Can you work these out from the model? Positions are in its coordinate system, mm. Face numbers are marked on the shaded views. A direction names the side the tool comes from. Coordinates: 2 decimals unless noted, no trailing zeros. Order: outer loops, then holes, each group sorted by start corner. A loop starts at its lowest first (then second) coordinate and runs counter-clockwise, first axis right, second up. Notation, with made-up numbers: (-31, 29.5) -> (-17, 29.5) arc R24 ccw to (-17, 47.5) -> close; hole circle Ø4 at (8.25, -23). An arc over 180 degrees is marked (long way). Return JSON: item names as keys, results as strings. Group by question number.
1) For pin 1 (1 mm diameter, centred on x = -7.5, y = -1.5, fed in from +Z); pin 2 (10 mm diameter, centred on x = -8.5, z = 5.5, fed in from -Y); pin 3 (9.5 mm diameter, centred on x = 2, y = 7, fed in from -Z); pin 4 (1 mm diameter, centred on y = 4, z = 8.5, fed in from +X), each with a flat end and sliding along its axis, tell me the tip position at first contact or that it passes through.
2) If I drill on probe 1 along Z at (x, y) = (-5, 11); probe 2 along Y at (x, z) = (0, 17.25); probe 3 along Y at (x, z) = (0, 2) (3 decimals), over which ranges is the centre line in solid material (lowest first)? Write a range as from..to.
3) If we section it at C-C, the plane z = 17.5: Please give me the cut outline in (x, y).
4) Thinking about a two-plate mould opening in X: for the marked faces 1, 2 and 3, which applies, +X half, -X half, draft (parallel to the pull), parting line (faces both ways), or undercut?
5) If we section it at A-A, the plane x = 0: Please give me the cut outline in (y, z) (3 decimals), then the cut area to 3 significant figures.
6) For the marked faces 4 and 5, which set-ups out of +Z, -Z, +X, -X, +Y, -Y let a thin tool reach every point of the face, with its end or its side?
7) If we section it at D-D, the plane y = 10.5: Please give me the cut outline in (x, z).
from build123d import *

# Parameters (mm, degrees)
F0_R     = 12.5
F1_DEPTH = 21.5
F2_R     = 15.85
F2_R_2   = 12.5
F3_DEPTH = 2
F5_D     = 15.75
F5_DEPTH = 23.5
F5_TIP   = 4.7317773748
F6_R     = 10
F7_DEPTH = 17
F8_W     = 1
F8_H     = 1.25


with BuildPart() as f1:
    # F0 (on Top) → F1 (new body)
    with BuildSketch(Plane.XY):
        Circle(F0_R)
    extrude(amount=F1_DEPTH)

    # F2 (on face) → F3 (join)
    with BuildSketch(Plane.XY.offset(21.5)):
        Circle(F2_R)
        Circle(F2_R_2, mode=Mode.SUBTRACT)
        Circle(F2_R_2)
    extrude(amount=F3_DEPTH)

    # F5
    with Locations(Plane.XY.offset(23.5)):
        with Locations((0, 0)):
            Hole(F5_D / 2, depth=F5_DEPTH)
            with Locations((0, 0, -(F5_DEPTH + F5_TIP / 2))):  # 118° drill point
                Cone(0, F5_D / 2, F5_TIP, mode=Mode.SUBTRACT)

    # F6 (on face) → F7 (cut)
    with BuildSketch(Plane.XY.offset(23.5)):
        Circle(F6_R)
    extrude(amount=-F7_DEPTH, mode=Mode.SUBTRACT)

    # F8 (on Front) → F9 (revolve, cut)
    with BuildSketch(Plane.XZ):
        with Locations((-12, 15.375)):
            Rectangle(F8_W, F8_H)
    revolve(axis=Axis((0, 0, 8), (0, 0, 1)), mode=Mode.SUBTRACT)


solid = f1.part
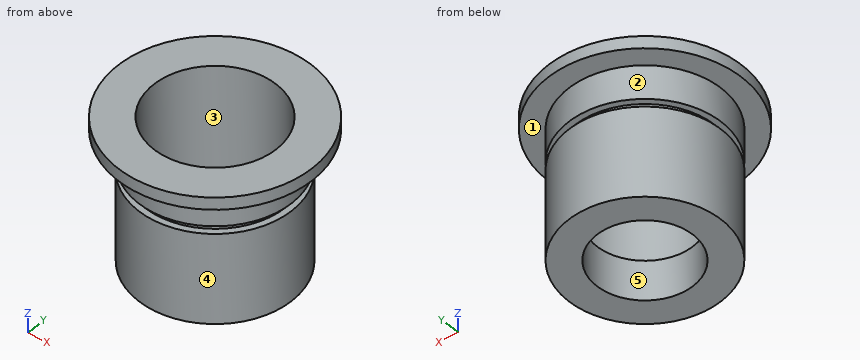
Result sheet:
{
 "1": {"pin 1": "stops at z = 6.5", "pin 2": "stops at y = -12", "pin 3": "stops at z = 0", "pin 4": "stops at x = 12"},
 "2": {"probe 1": "z = 0..14.75, 16..23.5", "probe 2": "y = -12.5..-10, 10..12.5", "probe 3": "y = -12.5..-7.875, 7.875..12.5"},
 "3": {"outline": "circle Ø25 at (0, 0); hole circle Ø20 at (0, 0)"},
 "4": {"face 1": "draft", "face 2": "parting line", "face 3": "undercut"},
 "5": {"outline": "(-15.85, 21.5) -> (-12.5, 21.5) -> (-12.5, 16) -> (-11.5, 16) -> (-11.5, 14.75) -> (-12.5, 14.75) -> (-12.5, 0) -> (-7.875, 0) -> (-7.875, 6.5) -> (-10, 6.5) -> (-10, 23.5) -> (-15.85, 23.5) -> close; (7.875, 0) -> (12.5, 0) -> (12.5, 14.75) -> (11.5, 14.75) -> (11.5, 16) -> (12.5, 16) -> (12.5, 21.5) -> (15.85, 21.5) -> (15.85, 23.5) -> (10, 23.5) -> (10, 6.5) -> (7.875, 6.5) -> close", "area": "156 mm2"},
 "6": {"face 4": "-Z", "face 5": "+Z, -Z"},
 "7": {"outline": "(-11.87, 21.5) -> (-6.78, 21.5) -> (-6.78, 16) -> (-4.69, 16) -> (-4.69, 14.75) -> (-6.78, 14.75) -> (-6.78, 0) -> (6.78, 0) -> (6.78, 14.75) -> (4.69, 14.75) -> (4.69, 16) -> (6.78, 16) -> (6.78, 21.5) -> (11.87, 21.5) -> (11.87, 23.5) -> (-11.87, 23.5) -> close"}
}
